Here's the drawing with two shaded views (mm, measured from the low corner). I have some questions. Coordinates: 2 decimals unless noted, no trailing zeros. Write each loop counter-clockwise with the first axis right and the second up, starting at its lowest first coordinate (ties: lowest second). Pieces come first, ordered by that corner, then holes.
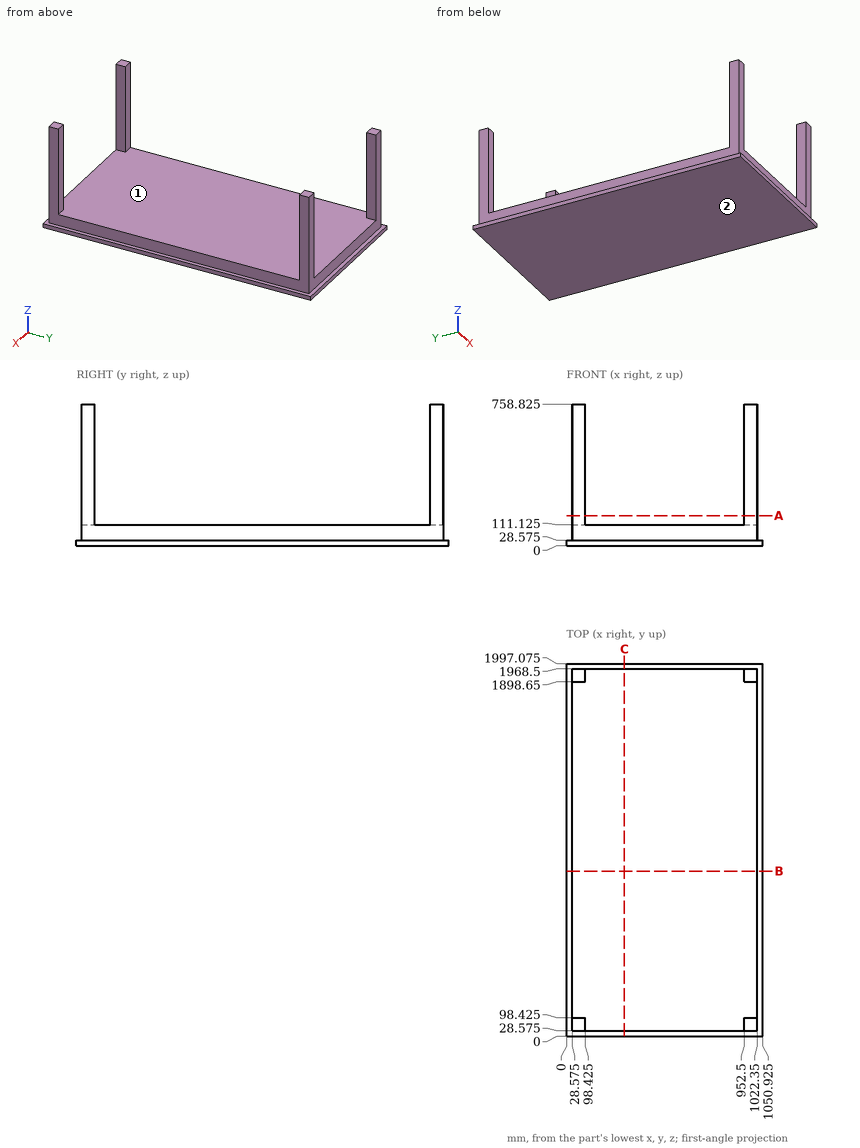
1. For pin 1 (21 mm diameter, centred on y = 80.5, z = 484.5, fed in from -X) (3 decimals); pin 2 (1.5 mm diameter, centred on x = 606.5, y = 1454, fed in from +Z) (3 decimals); pin 3 (4 mm diameter, centred on x = 340.5, y = 700.5, fed in from -Z); pin 4 (6 mm diameter, centred on x = 597, z = 99.5, fed in from -Y) (3 decimals), each with a flat end and sliding along its axis, tell me the tip position at first contact or that it passes through.
Verdict:
pin 1: stops at x = 28.575
pin 2: stops at z = 111.125
pin 3: stops at z = 0
pin 4: stops at y = 28.575
2. If we mould it in two halves opening along Y, with no side actions, what happens to the marked faces 1 and 2? For each: pulls with the +Y half, pulls with the -Y half, needs draft (parallel to the pull), parting line crosses it, or undercut.
Verdict:
face 1: undercut
face 2: needs draft
3. I want a section at B-B on y = 883.5. Please give me the cut outline in (x, z) (3 decimals), plus the area to 3 significant figures.
Verdict:
outline: (0, 0) - (1050.925, 0) - (1050.925, 28.575) - (1022.35, 28.575) - (1022.35, 111.125) - (28.575, 111.125) - (28.575, 28.575) - (0, 28.575) - close
area: 112,000 mm2
4. I want a section at A-A on z = 160. Please give me the cut outline in (x, y) (3 decimals), plus the area to 3 significant figures.
Verdict:
outline: (28.575, 28.575) - (98.425, 28.575) - (98.425, 98.425) - (28.575, 98.425) - close; (28.575, 1898.65) - (98.425, 1898.65) - (98.425, 1968.5) - (28.575, 1968.5) - close; (952.5, 28.575) - (1022.35, 28.575) - (1022.35, 98.425) - (952.5, 98.425) - close; (952.5, 1898.65) - (1022.35, 1898.65) - (1022.35, 1968.5) - (952.5, 1968.5) - close
area: 19,500 mm2
5. Please list where these lines run through material, in increasing order: line 1 along Y through (x, z) = (959, 257.5) (3 decimals); line 2 along Z through (x, y) = (443, 1430.5) (3 decimals); line 3 along X through (y, z) = (223, 104) (3 decimals).
Verdict:
line 1: y = 28.575 to 98.425, 1898.65 to 1968.5
line 2: z = 0 to 111.125
line 3: x = 28.575 to 1022.35
6. I want a section at C-C on x = 309. Please give me the cut outline in (y, z) (3 decimals).
Verdict:
outline: (0, 0) - (1997.075, 0) - (1997.075, 28.575) - (1968.5, 28.575) - (1968.5, 111.125) - (28.575, 111.125) - (28.575, 28.575) - (0, 28.575) - close
